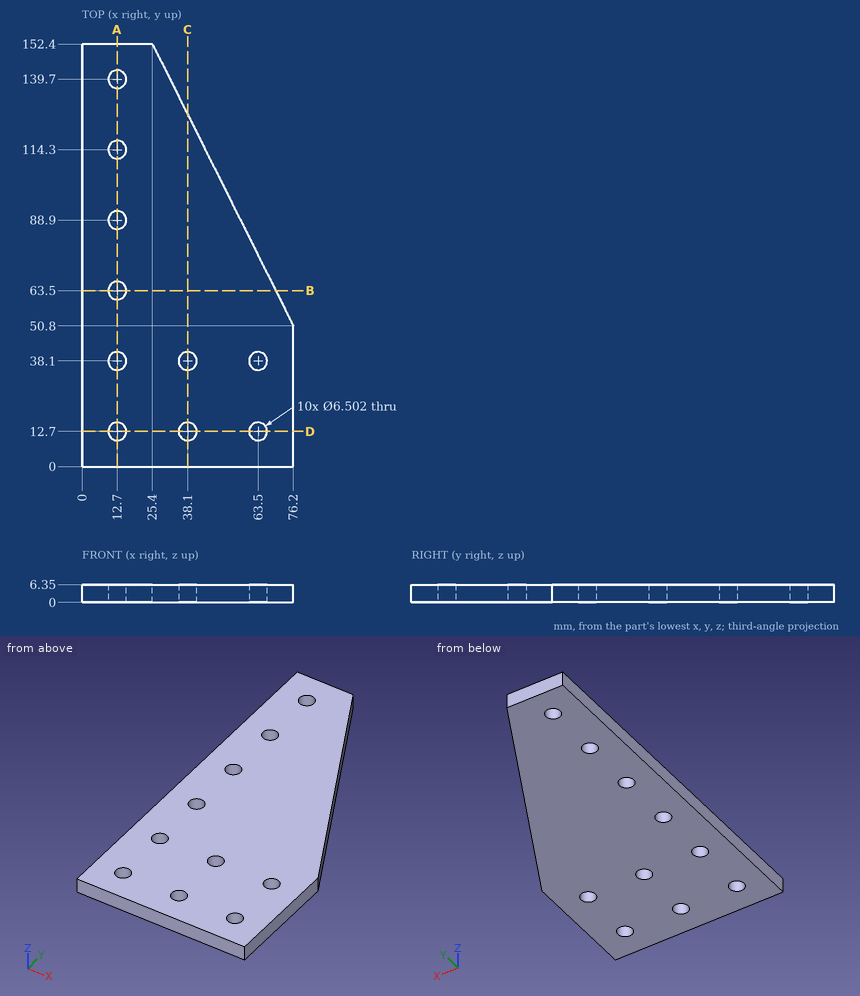
Input: dimensioned drawing with shaded views. Units: mm. Origin: part minimum x, y, z. Give positions to 0.01 mm unless a question says otherwise; leave off trailing zeros. Write each loop counter-clockwise with the first axis right and the second up, starting at its lowest first coordinate (ties: lowest second). Pieces come first, ordered by that corner, then holes. Notation, with made-up numbers: M 45,-39 L 74,-39 A19 ccw 74,-31 Z; hole C 35,-2 d2. An arc over 180 degrees is marked long. Return JSON: item names as keys, results as strings. Group by question number.
1) Cut plane B-B, the plane y = 63.5. Output: boundary loops of the cut face in (x, z).
2) Cut plane A-A, the plane x = 12.7. Output: boundary loops of the cut face in (y, z).
3) Material intervals for line 1 along X through (y, z) = (37, 2.5); line 2 along X through (y, z) = (145, 3.5); line 3 along Y through (x, z) = (26.5, 5), sorted ascending. Write a range as [from, to].
4) Cut plane D-D, the plane y = 12.7. Output: boundary loops of the cut face in (x, z).
5) Cut plane C-C, the plane x = 38.1. Output: boundary loops of the cut face in (y, z), plus the area to 3 significant figures.
Recorded:
{
 "1": {"outline": "M 0,0 L 9.45,0 L 9.45,6.35 L 0,6.35 Z; M 15.95,0 L 69.85,0 L 69.85,6.35 L 15.95,6.35 Z"},
 "2": {"outline": "M 0,0 L 9.45,0 L 9.45,6.35 L 0,6.35 Z; M 15.95,0 L 34.85,0 L 34.85,6.35 L 15.95,6.35 Z; M 41.35,0 L 60.25,0 L 60.25,6.35 L 41.35,6.35 Z; M 66.75,0 L 85.65,0 L 85.65,6.35 L 66.75,6.35 Z; M 92.15,0 L 111.05,0 L 111.05,6.35 L 92.15,6.35 Z; M 117.55,0 L 136.45,0 L 136.45,6.35 L 117.55,6.35 Z; M 142.95,0 L 152.4,0 L 152.4,6.35 L 142.95,6.35 Z"},
 "3": {"line 1": "x = [0, 9.64], [15.76, 35.04], [41.16, 60.44], [66.56, 76.2]", "line 2": "x = [0, 29.1]", "line 3": "y = [0, 150.2]"},
 "4": {"outline": "M 0,0 L 9.45,0 L 9.45,6.35 L 0,6.35 Z; M 15.95,0 L 34.85,0 L 34.85,6.35 L 15.95,6.35 Z; M 41.35,0 L 60.25,0 L 60.25,6.35 L 41.35,6.35 Z; M 66.75,0 L 76.2,0 L 76.2,6.35 L 66.75,6.35 Z"},
 "5": {"outline": "M 0,0 L 9.45,0 L 9.45,6.35 L 0,6.35 Z; M 15.95,0 L 34.85,0 L 34.85,6.35 L 15.95,6.35 Z; M 41.35,0 L 127,0 L 127,6.35 L 41.35,6.35 Z", "area": "724 mm²"}
}
